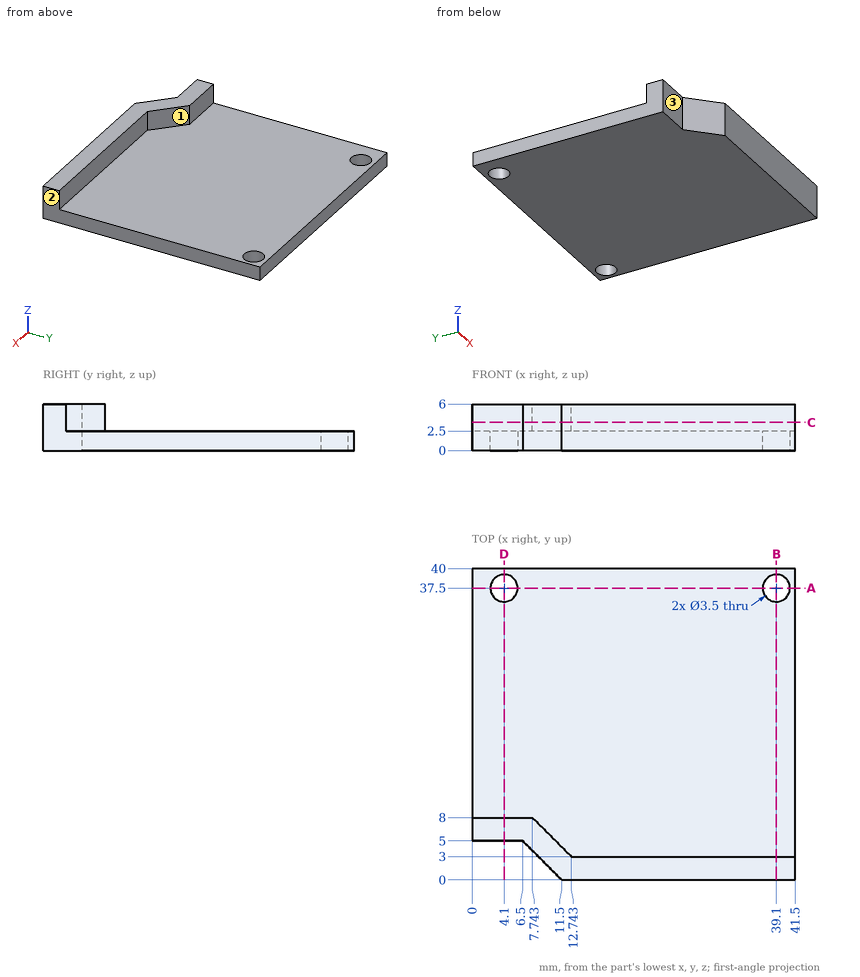
Geometry: see drawing. Coordinates: mm, zero at the bounding-box minimum. A direction names the side the tool comes from. Give positions to 0.01 mm unless a question says otherwise; leave off trailing zeros. Loops run counter-clockwise (first coordinate to the right, second up) from the corner with the lowest first, then second, coordinate; pieces in that order, holes last. Notation, with made-up numbers: (-27, 43.25) - (-9, 43.25) arc R26 ccw to (-9, 58.25) - close; hole circle Ø9 at (51, -24). An arc over 180 degrees is marked (long way). Use CSV: the item, a comma, the result in double quotes. Start each with the question number.
Item 1: Contact query for flat-ended pins moving along their axis: P1, Ø1.5, axis at x = 7.5, y = 17, coming from the +Z side; P2, Ø3, axis at x = 39.1, y = 37.5, coming from the +Z side; P3, Ø1, axis at x = 5.5, z = 3.5, coming from the +Y side; P4, Ø1.8, axis at x = 30.5, z = 3.5, coming from the +Y side. Output: stop coordinate, or through.
Item 2: Section B-B on x = 39.1. Return loops of the section in (y, z), then the cut area to 3 significant figures.
Item 3: Section D-D on x = 4.1. Return loops of the section in (y, z).
Item 4: Section C-C on z = 3.65. Return loops of the section in (x, y), then the cut area to 3 significant figures.
Item 5: Line query: line 1 (Y direction, x = 39.1, z = 0.85); line 2 (Y direction, x = 4.1, z = 1.7); line 3 (Y direction, x = 26, z = 5.4). Output: solid intervals per line, ascending.
Item 6: Reachability of the marked faces 1, 2 and 3 from +Z, -Z, +X, -X, +Y, -Y: full face, straight path, thin tool, end or side. Return the list, or none.
Item 7: Section A-A on y = 37.5. Return loops of the section in (x, z).
Ans:
1,P1,"stops at z = 2.5"
1,P2,"passes through"
1,P3,"stops at y = 8"
1,P4,"stops at y = 3"
2,outline,"(0, 0) - (35.75, 0) - (35.75, 2.5) - (3, 2.5) - (3, 6) - (0, 6) - close; (39.25, 0) - (40, 0) - (40, 2.5) - (39.25, 2.5) - close"
2,area,"102 mm2"
3,outline,"(5, 0) - (35.75, 0) - (35.75, 2.5) - (8, 2.5) - (8, 6) - (5, 6) - close; (39.25, 0) - (40, 0) - (40, 2.5) - (39.25, 2.5) - close"
4,outline,"(0, 5) - (6.5, 5) - (11.5, 0) - (41.5, 0) - (41.5, 3) - (12.74, 3) - (7.74, 8) - (0, 8) - close"
4,area,"131 mm2"
5,line 1,"y = 0 to 35.75, 39.25 to 40"
5,line 2,"y = 5 to 35.75, 39.25 to 40"
5,line 3,"y = 0 to 3"
6,face 1,"+Z, +X, +Y"
6,face 2,"+Z, -Z, +X, +Y, -Y"
6,face 3,"+Z, -Z, -X, -Y"
7,outline,"(0, 0) - (2.35, 0) - (2.35, 2.5) - (0, 2.5) - close; (5.85, 0) - (37.35, 0) - (37.35, 2.5) - (5.85, 2.5) - close; (40.85, 0) - (41.5, 0) - (41.5, 2.5) - (40.85, 2.5) - close"
